The listing builds one solid part. Answer for the finished solid, in the listing's coordinates (mm). Face numbers are marked on the shaded views. A direction names the side the tool comes from. Give positions to 0.01 mm unless a question says otherwise; leave off trailing zeros. Order: outer loops, then holes, each group sorted by start corner. A loop starts at its lowest first (then second) coordinate and runs counter-clockwise, first axis right, second up. Notation, with made-up numbers: (-15, 24) - (37, 24) arc R7 cw to (37, 34) - close; hole circle Ø3 at (54, 68.5). An arc over 180 degrees is marked (long way). Use CSV: the item, a comma, the result in double quotes.
```python
from build123d import *

# Parameters (mm, degrees)
PAD_DEPTH    = 2
PAD001_DEPTH = 5
PAD002_DEPTH = 23
PAD003_DEPTH = 4


with BuildPart() as part:
    # Sketch → Pad (new body)
    with BuildSketch(Plane.XZ):
        Polygon((5.9, 0), (4.9, 2), (4.9, 7.4), (0, 7.4), (0, 0), align=None)
    pad = extrude(amount=PAD_DEPTH)

    # Sketch001 → Pad001 (join)
    with BuildSketch(Plane.XZ.offset(2)):
        Polygon((5.9, 0), (4.9, 2), (4.9, 7.4), (3.35, 7.4), (3.35, 0), align=None)
    pad001 = extrude(amount=PAD001_DEPTH)

    # Sketch002 → Pad002 (join)
    with BuildSketch(Plane.XZ.offset(7)):
        Polygon((5.9, 0), (4.9, 2), (4.9, 7.4), (0, 7.4), (0, 5.4), (3.35, 5.4), (3.35, 0), align=None)
    pad002 = extrude(amount=PAD002_DEPTH)

    # Sketch003 → Pad003 (join)
    with BuildSketch(Plane.XZ.offset(30)):
        Polygon((5.9, 0), (4.9, 2), (4.9, 7.4), (0, 7.4), (0, 5.4), (2.2, 5.4), (2.2, 0), (3.35, 0), align=None)
    pad003 = extrude(amount=PAD003_DEPTH)

    # Mirrored: Pad, Pad001, Pad002, Pad003 across Sketch V_Axis
    add(pad.mirror(Plane(origin=(0, 0, 0), x_dir=(0, -1, 0), z_dir=(1, 0, 0))))
    add(pad001.mirror(Plane(origin=(0, 0, 0), x_dir=(0, -1, 0), z_dir=(1, 0, 0))))
    add(pad002.mirror(Plane(origin=(0, 0, 0), x_dir=(0, -1, 0), z_dir=(1, 0, 0))))
    add(pad003.mirror(Plane(origin=(0, 0, 0), x_dir=(0, -1, 0), z_dir=(1, 0, 0))))


solid = part.part
```
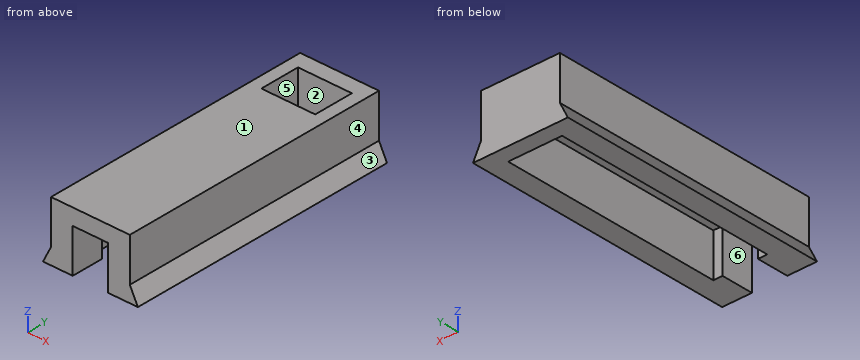
Item 1: Which of the six approach directions +Z, -Z, +X, -X, +Y, -Y give full straight-line access (tool end or side, diameter ignored) to the marked faces 4, 5 and 6?
Taken from the geometry:
face 4,"+Z, +X, +Y, -Y"
face 5,"-Z"
face 6,"-Z, -Y"
Item 2: The mould has two halves that part along X. Classify the marked faces 1, 2 and 3: +X half, -X half, draft (parallel to the pull), parting line (faces both ways), or undercut.
Taken from the geometry:
face 1,"draft"
face 2,"undercut"
face 3,"+X half"
Item 3: The part is cut by section D-D (y = -21). Give the vertices of the cut face in (x, z).
Taken from the geometry:
outline,"(-5.9, 0) - (-3.35, 0) - (-3.35, 5.4) - (3.35, 5.4) - (3.35, 0) - (5.9, 0) - (4.9, 2) - (4.9, 7.4) - (-4.9, 7.4) - (-4.9, 2) - close"
Item 4: The part is cut by section B-B (y = -4). Give the vertices of the cut face in (x, z).
Taken from the geometry:
outline,"(-5.9, 0) - (-3.35, 0) - (-3.35, 7.4) - (-4.9, 7.4) - (-4.9, 2) - close; (3.35, 0) - (5.9, 0) - (4.9, 2) - (4.9, 7.4) - (3.35, 7.4) - close"
Item 5: The part is cut by section A-A (x = -3). Give the vertices of the cut face in (y, z).
Taken from the geometry:
outline,"(-34, 0) - (-30, 0) - (-30, 5.4) - (-7, 5.4) - (-7, 7.4) - (-34, 7.4) - close; (-2, 0) - (0, 0) - (0, 7.4) - (-2, 7.4) - close"
Item 6: The part is cut by section C-C (z = 6.75). Give the vertices of the cut face in (x, y).
Taken from the geometry:
outline,"(-4.9, -34) - (4.9, -34) - (4.9, 0) - (-4.9, 0) - close; hole (-3.35, -7) - (3.35, -7) - (3.35, -2) - (-3.35, -2) - close"
Item 7: Each of these flat-tipped pins is pushed along its axis until it touches: pin 1 (3.5 mm diameter, centred on x = 1, y = -18, fed in from -Z); pin 2 (1 mm diameter, centred on y = -29, z = 4, fed in from +X); pin 3 (1.5 mm diameter, centred on x = -2.5, z = 2.5, fed in from +Y); pin 4 (1.2 mm diameter, centred on y = -31, z = 2, fed in from -X). Where does it stop, or does it pass through?
Taken from the geometry:
pin 1,"z = 5.4"
pin 2,"x = 4.9"
pin 3,"y = 0"
pin 4,"x = -5.2"
Item 8: Find the intervals of material crossed by line 1 along Y through (x, z) = (-3, 6.75); line 2 along X through (y, z) = (-15.5, 3.75); line 3 along Y through (x, z) = (-2.25, 5), in increasing order.
Taken from the geometry:
line 1,"-34 to -7, -2 to 0"
line 2,"-4.9 to -3.35, 3.35 to 4.9"
line 3,"-34 to -30, -2 to 0"
